The listing builds one solid part. Answer for the finished solid, in the listing's coordinates (mm). A direction names the side the tool comes from. Round coordinates to 2 decimals unless told otherwise and drop trailing zeros. Loops run counter-clockwise (first coordinate to the right, second up) from the corner with the lowest first, then second, coordinate; pieces in that order, holes last. Notation, with made-up numbers: M 61,-23 L 111,-23 A14 ccw 111,-2 Z; hole C -32.75,-34 d11. An arc over 180 degrees is marked long. Put each result on its own line as item: value. Start each with the question number.
(1) Section B-B, the plane x = 91.5 is taken. Determine the outline of the cut face in (y, z), then the cut area to 3 significant figures.
(2) Determine the mould class of faces 3 (the face through (-30, -3, 0)), 4 (the face through (-5.346, 0.616, -13.986)), 5 (the face through (100, 7.5, 0)) for opening direction Z: released by +Z, released by -Z, zero draft, split by the parting line, or undercut.
(3) Flat-ended cylindrical pins translate along their axes: P1, Ø5, axis at y = -44, z = -11, coming from the +X side; P2, Ø2, axis at y = -2, z = 1.5, coming from the -X side; P3, Ø2, axis at x = 100.5, y = 8.5, coming from the +Z side. Find the tip coordinate at first contact, or state that the pin passes through.
(4) Straight lines are drawn through the part: line 1 (X direction, y = -10, z = 2.25); line 2 (X direction, y = 6, z = 5.25); line 3 (X direction, y = 4.5, z = 9.5). For each, find the intervals that lie inside material, in ascending order.
(5) Section C-C, the plane x = 53 is taken. Determine the outline of the cut face in (y, z).
(6) Section A-A, the plane y = 0 is taken. Determine the outline of the cut face in (x, z).
(7) Which of the six approach directions +Z, -Z, +X, -X, +Y, -Y give full straight-line access (tool end or side, diameter ignored) to faces 1 (the face through (-13, 17, 0)), 2 (the face through (-15, 0, 0))?
```python
from build123d import *

# Parameters (mm, degrees)
SCHIZZO1_R                   = 9.5
ESTRUSIONE_ESTRUSIONE1_DEPTH = 120
TAGLIO_ESTRUSIONE1_START     = -40
TAGLIO_ESTRUSIONE1_DEPTH     = 40
SCHIZZO3_R                   = 14
ESTRUSIONE_ESTRUSIONE2_DEPTH = 14
ESTRUSIONE_ESTRUSIONE3_DEPTH = 10
SMUSSO1_SIZE                 = 5
SMUSSO2_SIZE                 = 2
SMUSSO3_SIZE                 = 5
SMUSSO4_SIZE                 = 0.5
ESTRUSIONE_ESTRUSIONE4_START = 9
SCHIZZO7_R                   = 8
SCHIZZO7_R_2                 = 5
ESTRUSIONE_ESTRUSIONE4_DEPTH = 9
SMUSSO5_SIZE                 = 0.5


# Some blends are built 0.0001 mm under size
with BuildPart() as part:
    # Schizzo1 → Estrusione-Estrusione1 (new body)
    with BuildSketch(Plane(origin=(0, 0, 0), x_dir=(0, 0, -1), z_dir=(1, 0, 0))):
        Circle(SCHIZZO1_R)
    extrude(amount=ESTRUSIONE_ESTRUSIONE1_DEPTH)

    # Schizzo2 → Taglio-Estrusione1 (cut)
    with BuildSketch(Plane(origin=(120, 0, 0), x_dir=(0, 0, -1), z_dir=(1, 0, 0)).offset(TAGLIO_ESTRUSIONE1_START)):
        with BuildLine():
            Line((-2, 9.287087811), (-2, 7.5))
            Line((-2, 7.5), (2, 7.5))
            Line((2, 7.5), (2, 9.287087811))
            ThreePointArc((2, 9.287087811), (0, 9.5), (-2, 9.287087811))
        make_face()
    extrude(amount=TAGLIO_ESTRUSIONE1_DEPTH, mode=Mode.SUBTRACT)

    # Schizzo3 → Estrusione-Estrusione2 (add)
    with BuildSketch(Plane.ZY):
        Circle(SCHIZZO3_R)
    extrude(amount=ESTRUSIONE_ESTRUSIONE2_DEPTH)

    # Schizzo4 → Estrusione-Estrusione3 (add, symmetric)
    with BuildSketch(Plane.XY):
        with BuildLine():
            Line((-10, 19), (-10, 9.5))
            Line((-10, 9.5), (-15, 9.5))
            Line((-15, 9.5), (-15, -9.5))
            Line((-15, -9.5), (-10, -9.5))
            Line((-10, -9.5), (-10, -19))
            ThreePointArc((-10, -19), (-10.681483474, -24.176380902), (-12.679491924, -29))
            Line((-12.679491924, -29), (-32.352250588, -63.074217531))
            Line((-32.352250588, -63.074217531), (-49.672758664, -53.074217531))
            Line((-49.672758664, -53.074217531), (-30, -19))
            Line((-30, -19), (-30, 19))
            Line((-30, 19), (-10, 19))
        make_face()
    extrude(amount=ESTRUSIONE_ESTRUSIONE3_DEPTH, both=True)

    # Smusso1
    smusso1_edges = [part.edges().sort_by_distance(p)[0] for p in [
        (-10, 19, 0),
        (-30, 19, 0),
    ]]
    chamfer(smusso1_edges, length=SMUSSO1_SIZE - 0.0001)  # a hair under: the kernel refuses the full size

    # Smusso2
    # the kernel refuses this chamfer: 2 mm, written as the material it adds along each edge
    with BuildSketch(Plane(origin=(-15, 9.5, 10), x_dir=(0.9996219169112968, 0.027495876610586487, 0), z_dir=(0, 0, -1)), Plane(origin=(-15, -9.5, 10), x_dir=(-0.02749587661058651, 0.9996219169112968, 0), z_dir=(0, 0, -1))) as smusso2_piece_1:
        Polygon((SMUSSO2_SIZE * 0.999621916911, SMUSSO2_SIZE * 0.0274958766106), (-SMUSSO2_SIZE * 0.0274958766106, SMUSSO2_SIZE * 0.999621916911), (0, 0), align=None)
    extrude(amount=20)

    # Smusso3
    smusso3_edges = [part.edges().sort_by_distance(p)[0] for p in [
        (-49.672758664, -53.074217531, 0),
        (-32.352250588, -63.074217531, 0),
    ]]
    chamfer(smusso3_edges, length=SMUSSO3_SIZE)

    # Schizzo6 → Taglia-Rivoluzione1 (revolve, cut)
    with BuildSketch(Plane.XY, mode=Mode.PRIVATE) as taglia_rivoluzione1_sk:
        Polygon((-43.172758664, -41.815887282), (-25.852250588, -51.815887282), (-23.352250588, -47.485760263), (-40.672758664, -37.485760263), align=None)
    revolve(taglia_rivoluzione1_sk.sketch.rotate(Axis((-115.6, 0, 0), (0.8660254037844387, -0.5000000000000001, 0)), 180), axis=Axis((-115.6, 0, 0), (0.8660254037844387, -0.5000000000000001, 0)), mode=Mode.SUBTRACT)

    # Smusso4
    smusso4_edges = [part.edges().sort_by_distance(p)[0] for p in [
        (-23.352250588, -47.485760263, 0),
    ]]
    chamfer(smusso4_edges, length=SMUSSO4_SIZE)

    # Schizzo7 → Estrusione-Estrusione4 (add)
    with BuildSketch(Plane(origin=(-14.272758664, 8.240381057, 0), x_dir=(0, 0, 1), z_dir=(-0.8660254037844383, 0.5000000000000009, 0)).offset(ESTRUSIONE_ESTRUSIONE4_START)):
        with Locations(Location((0, -57.8, 0), (0, 0, 270))):
            Circle(SCHIZZO7_R)
        with Locations(Location((0, -57.8, 0), (0, 0, 270))):
            Circle(SCHIZZO7_R_2, mode=Mode.SUBTRACT)
    extrude(amount=-ESTRUSIONE_ESTRUSIONE4_DEPTH)

    # Smusso5
    smusso5_edges = [part.edges().sort_by_distance(p)[0] for p in [
        (-48.466987298, -32.985760263, 0),
    ]]
    chamfer(smusso5_edges, length=SMUSSO5_SIZE)


solid = part.part
```
Recorded:
1. outline: M 7.5,-2 L 7.5,2 L 9.29,2 A9.5 ccw long 9.29,-2 Z
1. area: 276 mm²
2. face 3: zero draft
2. face 4: split by the parting line
2. face 5: undercut
3. P1: stops at x = -20.02
3. P2: stops at x = -30
3. P3: stops at z = 5.83
4. line 1: x = -30 to 0
4. line 2: x = -30 to -15, -14 to 120
4. line 3: x = -30 to -15, -14 to 0
5. outline: C 0,0 d19
6. outline: M -30,-10 L -15,-10 L -15,10 L -30,10 Z; M -14,-14 L 0,-14 L 0,-9.5 L 120,-9.5 L 120,9.5 L 0,9.5 L 0,14 L -14,14 Z
7. face 1: +Z, -Z, +X, +Y
7. face 2: +Z, -Z
